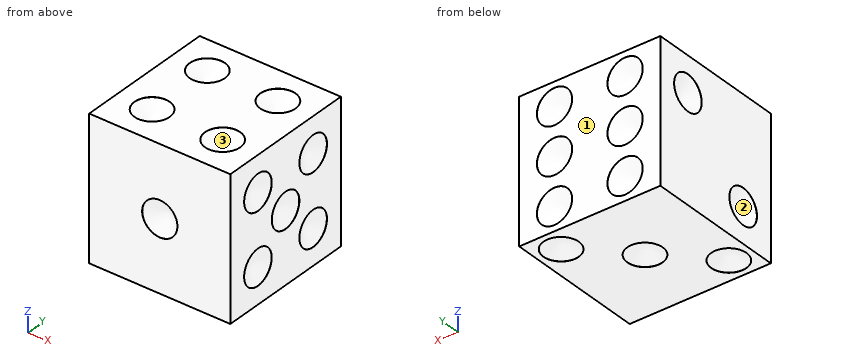
from build123d import *

# Parameters (mm, degrees)
F0_W          = 25.4
F0_H          = 25.4
F1_DEPTH      = 12.7
F1_DEPTH_BACK = 12.7
F3_D          = 6.35
F3_DEPTH      = 0.0254
F3_TIP        = 1.9077324654
F5_D          = 6.35
F5_DEPTH      = 0.0254
F5_TIP        = 1.9077324654
F7_D          = 6.35
F7_DEPTH      = 0.0254
F7_TIP        = 1.9077324654
F9_D          = 6.35
F9_DEPTH      = 0.0254
F9_TIP        = 1.9077324654
F11_D         = 6.35
F11_DEPTH     = 0.0254
F11_TIP       = 1.9077324654
F13_D         = 6.35
F13_DEPTH     = 0.0254
F13_TIP       = 1.9077324654


with BuildPart() as f1:
    # F0 (on Front) → F1 (new body, two sides)
    with BuildSketch(Plane.XZ) as f1_sk:
        with Locations((-12.7, 12.7)):
            Rectangle(F0_W, F0_H)
    extrude(amount=F1_DEPTH)
    extrude(f1_sk.sketch, amount=-F1_DEPTH_BACK)

    # F3
    with Locations(Plane.XZ.offset(12.7)):
        with Locations((-12.7, 12.7)):
            Hole(F3_D / 2, depth=F3_DEPTH)
            with Locations((0, 0, -(F3_DEPTH + F3_TIP / 2))):  # 118° drill point
                Cone(0, F3_D / 2, F3_TIP, mode=Mode.SUBTRACT)

    # F5
    with Locations(Plane.XY.offset(25.4)):
        with Locations((-19.05, 6.35), (-6.35, 6.35), (-6.35, -6.35), (-19.05, -6.35)):
            Hole(F5_D / 2, depth=F5_DEPTH)
            with Locations((0, 0, -(F5_DEPTH + F5_TIP / 2))):  # 118° drill point
                Cone(0, F5_D / 2, F5_TIP, mode=Mode.SUBTRACT)

    # F7
    with Locations(Plane(origin=(0, 0, 0), x_dir=(1, 0, 0), z_dir=(0, 0, -1))):
        with Locations((-21.1666666667, 8.4666666667), (-12.7, 0), (-4.2333333333, -8.4666666667)):
            Hole(F7_D / 2, depth=F7_DEPTH)
            with Locations((0, 0, -(F7_DEPTH + F7_TIP / 2))):  # 118° drill point
                Cone(0, F7_D / 2, F7_TIP, mode=Mode.SUBTRACT)

    # F9
    with Locations(Plane.YZ):
        with Locations((-6.35, 19.05), (0, 12.7), (6.35, 19.05), (6.35, 6.35), (-6.35, 6.35)):
            Hole(F9_D / 2, depth=F9_DEPTH)
            with Locations((0, 0, -(F9_DEPTH + F9_TIP / 2))):  # 118° drill point
                Cone(0, F9_D / 2, F9_TIP, mode=Mode.SUBTRACT)

    # F11
    with Locations(Plane(origin=(-25.4, 0, 0), x_dir=(0, -1, 0), z_dir=(-1, 0, 0))):
        with Locations((-6.35, 19.05), (6.35, 6.35)):
            Hole(F11_D / 2, depth=F11_DEPTH)
            with Locations((0, 0, -(F11_DEPTH + F11_TIP / 2))):  # 118° drill point
                Cone(0, F11_D / 2, F11_TIP, mode=Mode.SUBTRACT)

    # F13
    with Locations(Plane(origin=(0, 12.7, 0), x_dir=(-1, 0, 0), z_dir=(0, 1, 0))):
        with Locations((6.35, 21.1666666667), (6.35, 12.7), (6.35, 4.2333333333), (19.05, 21.1666666667), (19.05, 12.7), (19.05, 4.2333333333)):
            Hole(F13_D / 2, depth=F13_DEPTH)
            with Locations((0, 0, -(F13_DEPTH + F13_TIP / 2))):  # 118° drill point
                Cone(0, F13_D / 2, F13_TIP, mode=Mode.SUBTRACT)


solid = f1.part
Source: CAD feature listing. Evaluate the final solid. Frame: model axes, mm. Face numbers are marked on the shaded views. Give positions to 0.01 mm unless a question says otherwise; leave off trailing zeros. Write item = value, one per line. Start each with the question number.
Q1. Pin query (flat end, axial travel): pin 1 Ø1 at (y, z) = (6, 18.5) entering from +X; pin 2 Ø5 at (x, z) = (-19.05, 12.7) entering from +Y; pin 3 Ø5 at (y, z) = (6.35, 6.35) entering from +X. Return the tip coordinate at first contact, or that it passes through.
Q2. Cut plane A-A, the plane y = 11.25. Give the number of separate pieces and of enclosed holes in the cut face, then the cut area to 3 significant figures.
Q3. Draft query along Z for the marked faces 1, 2 and 3. Return one class per face: +Z half, -Z half, draft (parallel to the pull), parting line (faces both ways), or undercut.
Q4. Material intervals for probe 1 along Y at (x, z) = (-1.75, 6.25); probe 2 along X at (y, z) = (-7, 17.75); probe 3 along Y at (x, z) = (-5.5, 20), sorted ascending.
Computed values:
q1.pin_1 = -1.24
q1.pin_2 = 12.27
q1.pin_3 = -0.43
q2.separate_pieces = 1
q2.enclosed_holes = 6
q2.area = 632 mm²
q3.face_1 = draft
q3.face_2 = undercut
q3.face_3 = +Z half
q4.probe_1 = -12.7 to -6.64, -6.06 to 6.06, 6.64 to 12.7
q4.probe_2 = -25.4 to -1.06
q4.probe_3 = -12.7 to 11.63
